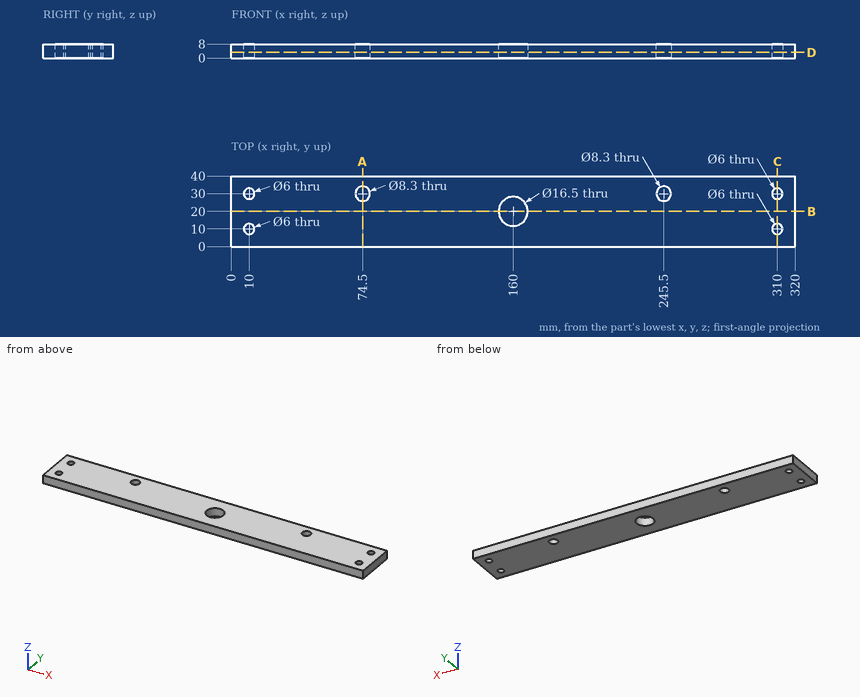
Print and shaded views of the part. All mm, measured from the part's lowest x, y and z. Round coordinates to 2 decimals unless told otherwise and drop trailing zeros. Write each loop counter-clockwise with the first axis right and the second up, starting at its lowest first coordinate (ties: lowest second). Pieces come first, ordered by that corner, then holes. Notation, with made-up numbers: (82.5, 52.25) -> (122.5, 52.25) arc R25 ccw to (122.5, 66.25) -> close; hole circle Ø5 at (-35.75, 14.5). An arc over 180 degrees is marked (long way). Answer in a Markdown table with one row per item. Add a question column.
Item 1: Saw through at B-B, the plane y = 20. Write the cut outline in (x, z), then the cut area to 3 significant figures.
Item 2: Saw through at A-A, the plane x = 74.5. Write the cut outline in (y, z), then the cut area to 3 significant figures.
Item 3: Saw through at C-C, the plane x = 310. Write the cut outline in (y, z).
Item 4: Drill centre lines: line 1 (Y direction, x = 310, z = 2.25); line 2 (Y direction, x = 74.5, z = 4.75); line 3 (X direction, y = 19, z = 4). Where is each one in solid material? Low to high. Write a range as from..to.
Item 5: Saw through at D-D, the plane z = 3.25. Write the cut outline in (x, y).
Findings below:
| question | item | result |
|---|---|---|
| 1 | outline | (0, 0) -> (151.75, 0) -> (151.75, 8) -> (0, 8) -> close; (168.25, 0) -> (320, 0) -> (320, 8) -> (168.25, 8) -> close |
| 1 | area | 2,430 mm^2 |
| 2 | outline | (0, 0) -> (25.85, 0) -> (25.85, 8) -> (0, 8) -> close; (34.15, 0) -> (40, 0) -> (40, 8) -> (34.15, 8) -> close |
| 2 | area | 254 mm^2 |
| 3 | outline | (0, 0) -> (7, 0) -> (7, 8) -> (0, 8) -> close; (13, 0) -> (27, 0) -> (27, 8) -> (13, 8) -> close; (33, 0) -> (40, 0) -> (40, 8) -> (33, 8) -> close |
| 4 | line 1 | y = 0..7, 13..27, 33..40 |
| 4 | line 2 | y = 0..25.85, 34.15..40 |
| 4 | line 3 | x = 0..151.81, 168.19..320 |
| 5 | outline | (0, 0) -> (320, 0) -> (320, 40) -> (0, 40) -> close; hole circle Ø6 at (10, 10); hole circle Ø6 at (10, 30); hole circle Ø8.3 at (74.5, 30); hole circle Ø16.5 at (160, 20); hole circle Ø8.3 at (245.5, 30); hole circle Ø6 at (310, 10); hole circle Ø6 at (310, 30) |
